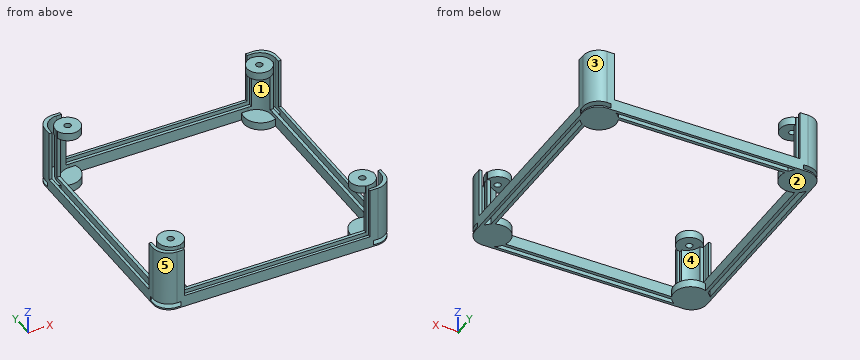
```python
from build123d import *

# Parameters (mm, degrees)
SKETCH1_R             = 11
BOSS_EXTRUDE1_DEPTH   = 5
BOSS_EXTRUDE1_2_DEPTH = 5
BOSS_EXTRUDE1_3_DEPTH = 5
BOSS_EXTRUDE1_4_DEPTH = 5
BOSS_EXTRUDE2_START   = 1
BOSS_EXTRUDE2_DEPTH   = 3
BOSS_EXTRUDE2_2_DEPTH = 3
BOSS_EXTRUDE2_3_DEPTH = 3
BOSS_EXTRUDE2_4_DEPTH = 3
SKETCH3_W             = 150
SKETCH3_H             = 150
SKETCH3_W_2           = 146.352390556
SKETCH3_H_2           = 146.352390556
BOSS_EXTRUDE4_DEPTH   = 40
SKETCH3_W_3           = 140.198704382
SKETCH3_H_3           = 140.198704382
SKETCH3_W_4           = 136
SKETCH3_H_4           = 136
BOSS_EXTRUDE4_2_DEPTH = 40
FILLET1_R             = 10
FILLET2_R             = 10
BOSS_EXTRUDE6_START   = 40
SKETCH6_W             = 120
SKETCH6_H             = 120
SKETCH6_H_2           = 23.888569694
SKETCH6_W_2           = 20.217809466
BOSS_EXTRUDE6_DEPTH   = 32.5
SKETCH7_R             = 8
SKETCH7_R_2           = 2.14
BOSS_EXTRUDE7_DEPTH   = 5


with BuildPart() as part:
    # Sketch1 → Boss-Extrude1 (new body)
    with BuildSketch(Plane.XY):
        with Locations((-64, -64)):
            Circle(SKETCH1_R)
    extrude(amount=BOSS_EXTRUDE1_DEPTH)


with BuildPart() as body_2:
    # Sketch1 → Boss-Extrude1 2 (new body)
    with BuildSketch(Plane.XY):
        with Locations((-64, 64)):
            Circle(SKETCH1_R)
    extrude(amount=BOSS_EXTRUDE1_2_DEPTH)


with BuildPart() as body_3:
    # Sketch1 → Boss-Extrude1 3 (new body)
    with BuildSketch(Plane.XY):
        with Locations((64, -64)):
            Circle(SKETCH1_R)
    extrude(amount=BOSS_EXTRUDE1_3_DEPTH)


with BuildPart() as body_4:
    # Sketch1 → Boss-Extrude1 4 (new body)
    with BuildSketch(Plane.XY):
        with Locations((64, 64)):
            Circle(SKETCH1_R)
    extrude(amount=BOSS_EXTRUDE1_4_DEPTH)


with BuildPart() as body_5:
    # Sketch2 → Boss-Extrude2 (new body)
    with BuildSketch(Plane.XY.offset(BOSS_EXTRUDE2_START)):
        with BuildLine():
            Line((-57.636038969, -70.363961031), (-77.792434068, -90.52035613))
            ThreePointArc((-77.792434068, -90.52035613), (-90.52035613, -90.52035613), (-90.52035613, -77.792434068))
            Line((-90.52035613, -77.792434068), (-70.363961031, -57.636038969))
            ThreePointArc((-70.363961031, -57.636038969), (-57.636038969, -57.636038969), (-57.636038969, -70.363961031))
        make_face()
    extrude(amount=BOSS_EXTRUDE2_DEPTH)


with BuildPart() as body_6:
    # Sketch2 → Boss-Extrude2 2 (new body)
    with BuildSketch(Plane.XY.offset(BOSS_EXTRUDE2_START)):
        with BuildLine():
            Line((-70.363961031, 57.636038969), (-87.555608123, 74.827686061))
            ThreePointArc((-87.555608123, 74.827686061), (-87.555608123, 87.555608123), (-74.827686061, 87.555608123))
            Line((-74.827686061, 87.555608123), (-57.636038969, 70.363961031))
            ThreePointArc((-57.636038969, 70.363961031), (-57.636038969, 57.636038969), (-70.363961031, 57.636038969))
        make_face()
    extrude(amount=BOSS_EXTRUDE2_2_DEPTH)


with BuildPart() as body_7:
    # Sketch2 → Boss-Extrude2 3 (new body)
    with BuildSketch(Plane.XY.offset(BOSS_EXTRUDE2_START)):
        with BuildLine():
            Line((70.363961031, -57.636038969), (87.260513721, -74.532591659))
            ThreePointArc((87.260513721, -74.532591659), (87.260513721, -87.260513721), (74.532591659, -87.260513721))
            Line((74.532591659, -87.260513721), (57.636038969, -70.363961031))
            ThreePointArc((57.636038969, -70.363961031), (57.636038969, -57.636038969), (70.363961031, -57.636038969))
        make_face()
    extrude(amount=BOSS_EXTRUDE2_3_DEPTH)


with BuildPart() as body_8:
    # Sketch2 → Boss-Extrude2 4 (new body)
    with BuildSketch(Plane.XY.offset(BOSS_EXTRUDE2_START)):
        with BuildLine():
            Line((57.636038969, 70.363961031), (76.733324594, 89.461246655))
            ThreePointArc((76.733324594, 89.461246655), (89.461246655, 89.461246655), (89.461246655, 76.733324594))
            Line((89.461246655, 76.733324594), (70.363961031, 57.636038969))
            ThreePointArc((70.363961031, 57.636038969), (57.636038969, 57.636038969), (57.636038969, 70.363961031))
        make_face()
    extrude(amount=BOSS_EXTRUDE2_4_DEPTH)


with BuildPart() as body_9:
    # Sketch3 → Boss-Extrude4 (new body)
    with BuildSketch(Plane.XY):
        Rectangle(SKETCH3_W, SKETCH3_H)
        Rectangle(SKETCH3_W_2, SKETCH3_H_2, mode=Mode.SUBTRACT)
    extrude(amount=BOSS_EXTRUDE4_DEPTH)

    # Fillet1
    fillet1_edges = [body_9.edges().sort_by_distance(p)[0] for p in [
        (-75, -75, 20),
        (-75, 75, 20),
        (75, 75, 20),
        (75, -75, 20),
        (-73.176195278, -73.176195278, 20),
        (73.176195278, -73.176195278, 20),
        (73.176195278, 73.176195278, 20),
        (-73.176195278, 73.176195278, 20),
    ]]
    fillet(fillet1_edges, radius=FILLET1_R)


with BuildPart() as body_10:
    # Sketch3 → Boss-Extrude4 2 (new body)
    with BuildSketch(Plane.XY):
        Rectangle(SKETCH3_W_3, SKETCH3_H_3)
        Rectangle(SKETCH3_W_4, SKETCH3_H_4, mode=Mode.SUBTRACT)
    extrude(amount=BOSS_EXTRUDE4_2_DEPTH)

    # Fillet2
    fillet2_edges = [body_10.edges().sort_by_distance(p)[0] for p in [
        (70.099352191, 70.099352191, 20),
        (70.099352191, -70.099352191, 20),
        (-70.099352191, -70.099352191, 20),
        (-70.099352191, 70.099352191, 20),
        (-68, -68, 20),
        (68, -68, 20),
        (68, 68, 20),
        (-68, 68, 20),
    ]]
    fillet(fillet2_edges, radius=FILLET2_R)


with BuildPart() as part_1:
    add(part.part)

    # Combine4: union body 4, body 3, body 2, body 9, body 10
    add(body_4.part)
    add(body_3.part)
    add(body_2.part)
    add(body_9.part)
    add(body_10.part)

    # Combine8: cut body 7, body 5, body 6, body 8
    add(body_7.part, mode=Mode.SUBTRACT)
    add(body_5.part, mode=Mode.SUBTRACT)
    add(body_6.part, mode=Mode.SUBTRACT)
    add(body_8.part, mode=Mode.SUBTRACT)


with BuildPart() as body_2_2:
    # Sketch6 → Boss-Extrude6 (new body)
    with BuildSketch(Plane.XY.offset(BOSS_EXTRUDE6_START)):
        Rectangle(SKETCH6_W, SKETCH6_H)
        with Locations((0, -71.944284847)):
            Rectangle(SKETCH6_W, SKETCH6_H_2)
        with Locations((-70.108904733, 0)):
            Rectangle(SKETCH6_W_2, SKETCH6_H)
        with Locations((0, 71.944284847)):
            Rectangle(SKETCH6_W, SKETCH6_H_2)
        with Locations((70.108904733, 0)):
            Rectangle(SKETCH6_W_2, SKETCH6_H)
    extrude(amount=-BOSS_EXTRUDE6_DEPTH)


with BuildPart() as part_2:
    add(part_1.part)

    # Combine9: cut body 2 2
    add(body_2_2.part, mode=Mode.SUBTRACT)

    # Sketch7 → Boss-Extrude7 (add)
    with BuildSketch(Plane.XY.offset(40)):
        with Locations((-62, -62)):
            Circle(SKETCH7_R)
        with Locations((-62, -62)):
            Circle(SKETCH7_R_2, mode=Mode.SUBTRACT)
        with Locations((-62, 62)):
            Circle(SKETCH7_R)
        with Locations((-62, 62)):
            Circle(SKETCH7_R_2, mode=Mode.SUBTRACT)
        with Locations((62, -62)):
            Circle(SKETCH7_R)
        with Locations((62, -62)):
            Circle(SKETCH7_R_2, mode=Mode.SUBTRACT)
        with Locations((62, 62)):
            Circle(SKETCH7_R)
        with Locations((62, 62)):
            Circle(SKETCH7_R_2, mode=Mode.SUBTRACT)
    extrude(amount=-BOSS_EXTRUDE7_DEPTH)


solid = part_2.part
```
Could you check a few things on this model? Use its own coordinates, in mm. Face numbers are marked on the shaded views. A direction names the side the tool comes from. Round coordinates to 2 decimals unless told otherwise and drop trailing zeros. Loops run counter-clockwise (first coordinate to the right, second up) from the corner with the lowest first, then second, coordinate; pieces in that order, holes last.
Q1. I want a section at C-C (z = 22). Give the number of separate pieces and of enclosed holes in the cut face, and give its area (3 significant figures).
Q2. I want a section at A-A (x = 18). Write out the boundary of the cut face in (y, z), and give its area (3 significant figures).
Q3. Thinking about a two-plate mould opening in X: for the marked faces 1, 2 and 3, which applies, pulls with the +X half, pulls with the -X half, needs draft (parallel to the pull), parting line crosses it, or undercut?
Q4. Please list where these lines run through material, in increasing order: L1, parallel to X at y = 4, z = 2.5; L2, parallel to Y at x = -62, z = 38.1.
Q5. On a 3-axis mill with a long thin cutter (end or side, diameter ignored), from which of +Z, -Z, +X, -X, +Y, -Y can I reach the whole of each face in a straight line? I mean the marked faces 4 and 5. Say none if no direction works.
Q6. For P1, Ø0.9, axis at x = 13, y = 74, coming from the +Z side; P2, Ø16.5, axis at x = -64, y = -61.5, coming from the +Z side; P3, Ø1.8, axis at y = 69, z = 31, coming from the +X side; P4, Ø2.5, axis at y = 69, z = 19, coming from the -X side, each with a flat end and sliding along its axis, tell me the tip position at first contact or that it passes through.
Answer below:
1. separate pieces: 8
1. enclosed holes: 0
1. area: 356 mm2
2. outline: (-75, 0) - (-73.18, 0) - (-73.18, 7.5) - (-75, 7.5) - close; (-70.1, 0) - (-68, 0) - (-68, 7.5) - (-70.1, 7.5) - close; (68, 0) - (70.1, 0) - (70.1, 7.5) - (68, 7.5) - close; (73.18, 0) - (75, 0) - (75, 7.5) - (73.18, 7.5) - close
2. area: 58.8 mm2
3. face 1: undercut
3. face 2: needs draft
3. face 3: pulls with the +X half
4. L1: x = -75 to -73.18, -70.1 to -68, 68 to 70.1, 73.18 to 75
4. L2: y = -75 to -73.18, -70 to -64.14, -59.86 to -54, 54 to 59.86, 64.14 to 70, 73.18 to 75
5. face 4: none
5. face 5: +Z, -Z, -X, -Y
6. P1: stops at z = 7.5
6. P2: stops at z = 40
6. P3: stops at x = 74.51
6. P4: stops at x = -74.61
